Autodesk Inventor part; units mm, degrees
sketch "Sketch1" plane through (0, 0, 0) normal (0, 0, 1) x (1, 0, 0)
  line L0 (0, 0) -> (25, 0)
  line L1 (25, 0) -> (25, 36)
  line L2 (25, 36) -> (0, 36)
  line L3 (0, 36) -> (0, 0)
  dimension "d0" = 25
  dimension "d1" = 36
extrude "Extrusion1" add sketch "Sketch1" along normal blind 6
sketch "Sketch2" plane through (0, 0, 0) normal (-1, 0, 0) x (0, 0, 1)
  line L0 (0, 0) -> (6, 0)
  line L1 (0, 36) -> (6, 36)
  line L2 (2.495, 0) -> (3.505, 0)
  line L3 (3.505, 0) -> (3.505, 36)
  line L4 (3.505, 36) -> (2.495, 36)
  line L5 (2.495, 36) -> (2.495, 0)
  point P0 (3, 0)
  point P1 (3, 0)
  dimension "d4" = 0
  dimension "d5" = 1.01
extrude "Extrusion2" cut sketch "Sketch2" against normal blind 6
sketch "Sketch3" plane through (25, 0, 0) normal (1, 0, 0) x (0, 0, -1)
  line L0 (0, 36) -> (-6, 36)
  line L1 (-3.505, 4.95) -> (-2.495, 4.95)
  line L2 (-2.495, 4.95) -> (-2.495, 31.05)
  line L3 (0, 0) -> (-6, 0)
  line L4 (0, 0) -> (0, 36)
  line L5 (-3.505, 4.95) -> (-3.505, 31.05)
  line L6 (-3.505, 31.05) -> (-2.495, 31.05)
  point P0 (-3.505, 0)
  point P1 (-2.495, 0)
  point P2 (-3, 4.95)
  point P3 (-3, 0)
  point P4 (0, 18)
  point P5 (-2.495, 18)
  dimension "d11" = 26.1
  dimension "d13" = 0
  dimension "d14" = 0
  dimension "d15" = 1.01
extrude "Extrusion3" cut sketch "Sketch3" against normal blind 18
sketch "Sketch4" plane through (25, 0, 0) normal (1, 0, 0) x (0, 0, -1)
  line L0 (0, 36) -> (0, 0)
  line L1 (-6, 36) -> (-6, 0)
  line L2 (0, 5.55) -> (-6, 5.55)
  line L3 (-6, 5.55) -> (-6, 30.45)
  line L4 (-6, 30.45) -> (0, 30.45)
  line L5 (0, 30.45) -> (0, 5.55)
  line L6 (-2.495, 4.95) -> (-3.505, 4.95)
  point P0 (0, 18)
  point P1 (0, 18)
  dimension "d16" = 0
  dimension "d19" = 0.6
extrude "Extrusion4" cut sketch "Sketch4" against normal blind 18
properties part number "camera_support_on_carbon_blade"
Geometry check sheet. Reference: the model listing, model coordinates, mm. A direction names the side the tool comes from. Give positions to 0.01 mm unless a question says otherwise; leave off trailing zeros. Order: outer loops, then holes, each group sorted by start corner. A loop starts at its lowest first (then second) coordinate and runs counter-clockwise, first axis right, second up.
1. Access from +Z, -Z, +X, -X, +Y, -Y to the whole of each face (thin tool, end or side, straight path). Record for faces 1 (the face through (16, 30.45, 1)), 2 (the face through (6, 18, 3)), 3 (the face through (16, 4.95, 3)), 4 (the face through (13, 36, 3)).
2. Release check for a two-part mould opening along Z. For faces 5 (the face through (3, 18, 3.505)), 6 (the face through (12, 0, 3)), 7 (the face through (16, 31.05, 3)), 8 (the face through (6.8, 18.3, 0)) record: pulls with the +Z half, pulls with the -Z half, needs draft (parallel to the pull), parting line crosses it, or undercut.
3. Thickness scan on L1, parallel to Z at x = 16, y = 5.5 (3 decimals); L2, parallel to Y at x = 20, z = 4.4; L3, parallel to X at y = 25, z = 0.6. Record the ranges inside material, lowest first.
4. Section check B-B, the plane z = 2.9. Enter the section's corners in (x, y), and give its area (3 significant figures).
5. Section check C-C, the plane y = 17. Enter the section's corners in (x, z) (3 decimals).
6. Section check A-A, the plane x = 10.5. Enter the section's corners in (y, z) (3 decimals), and give its area (3 significant figures).
7. Gauge pin test, flat ends, axial feed: pin 1 Ø0.5 at (y, z) = (12.5, 3) entering from -X; pin 2 Ø12 at (x, y) = (16, 23) entering from +Z. Record the tip position at first contact, or that the pin passes through.
Values follow:
1. face 1: +Z, -Z, +X
1. face 2: -X, +Y, -Y
1. face 3: +X
1. face 4: +Z, -Z, +X, -X, +Y
2. face 5: undercut
2. face 6: needs draft
2. face 7: undercut
2. face 8: pulls with the -Z half
3. L1: z = 0 to 2.495, 3.505 to 6
3. L2: y = 0 to 5.55, 30.45 to 36
3. L3: x = 0 to 7
4. outline: (6, 0) - (25, 0) - (25, 4.95) - (7, 4.95) - (7, 31.05) - (25, 31.05) - (25, 36) - (6, 36) - close
4. area: 214 mm2
5. outline: (0, 0) - (7, 0) - (7, 6) - (0, 6) - (0, 3.505) - (6, 3.505) - (6, 2.495) - (0, 2.495) - close
6. outline: (0, 0) - (5.55, 0) - (5.55, 2.495) - (4.95, 2.495) - (4.95, 3.505) - (5.55, 3.505) - (5.55, 6) - (0, 6) - close; (30.45, 0) - (36, 0) - (36, 6) - (30.45, 6) - (30.45, 3.505) - (31.05, 3.505) - (31.05, 2.495) - (30.45, 2.495) - close
6. area: 65.4 mm2
7. pin 1: stops at x = 6
7. pin 2: passes through
